Design review of the part built by this model. Coordinates are the model's own, in mm. A direction names the side the tool comes from. Round coordinates to 2 decimals unless told otherwise and drop trailing zeros. Write each loop counter-clockwise with the first axis right and the second up, starting at its lowest first coordinate (ties: lowest second). Pieces come first, ordered by that corner, then holes. Notation, with made-up numbers: (88.25, 48) -> (121.25, 48) arc R19 ccw to (121.25, 57) -> close; hole circle Ø1 at (68, -25). An arc over 180 degrees is marked (long way). One line per question, with ' | ' between items. Start each with the question number.
1) For faces 1 (the flat face through (3.549, 6.034, 2.875)), 2 (the flat face through (5, -2, 0)), 3 (the cylindrical face through (1.322, 4.197, 17.245)), 4 (the cylindrical face through (6.84, -0.9, 18.58)), 5 (the conical face through (-0.158, -7.184, 0.322)), list the 3-axis set-ups (+Z, -Z, +X, -X, +Y, -Y) from which the entire face can be reached by the end or side of a thin tool; tool diameter is ignored.
2) For probe 1 along X at (y, z) = (0, 6.5); probe 2 along X at (y, z) = (-1.25, 7); probe 3 along Y at (x, z) = (-0.75, -2), list the stretches that pass through material, from the lowest coordinate up.
3) Consider section A-A (z = 0.75). Give the boundary of the cut face in (x, y), then the cut area to 3 significant figures.
4) Mouldability with a two-part tool opening along X and no side actions: class faces 6 (the conical face through (0.158, 7.184, 0.322)), 7 (the flat face through (3.45, -6.09, 2.88)), 8 (the flat face through (-2, 3, -8)), 9 (the cylindrical face through (0, -3, -1)) as +X half, -X half, draft (parallel to the pull), parting line (faces both ways), or undercut.
5) Insertion check: pin 1 Ø3 at (x, z) = (-1.5, 16) entering from -Y; pin 2 Ø3.5 at (x, y) = (1, -1.5) entering from +Z; pin 3 Ø4 at (x, z) = (-4.5, 3.5) entering from +Y. Each pin has a flat end and moves straight along its axis. Give the tip position at first contact, or say it passes through.
Autodesk Inventor part; units mm, degrees
ref_plane "ANBAU_XY" through (0, 0, -4) normal (0, 0, 1) x (1, 0, 0)
ref_plane "ANBAU_YZ" through (0, 0, -4) normal (1, 0, 0) x (0, 1, 0)
ref_plane "ANBAU_ZX" through (0, 0, -4) normal (0, 1, 0) x (0, 0, 1)
sketch "Sketch_2" plane through (0, 0, 0) normal (1, 0, 0) x (0, 1, 0)
  line L0 (0, 0) -> (0, 19.9)
  line L1 (0, 19.9) -> (4.3, 19.9)
  line L2 (4.3, 19.9) -> (6.7347, 19.4707)
  arc A0 (6.9, 19.2737) -> (6.7347, 19.4707) centre (6.7, 19.2737) ccw
  line L3 (6.9, 19.2737) -> (6.9, 17.9)
  line L4 (6.9, 17.9) -> (4.7, 17.9)
  arc A1 (4.7, 17.9) -> (4.4, 17.6) centre (4.7, 17.6) ccw
  line L5 (4.4, 17.6) -> (4.4, 16.9)
  line L6 (4.4, 16.9) -> (5.7, 16.9)
  line L7 (5.7, 16.9) -> (5.9, 16.7)
  line L8 (5.9, 16.7) -> (5.9, 16)
  line L9 (5.9, 16) -> (5.8, 15.9)
  line L10 (5.8, 15.9) -> (5.9, 15.8)
  line L11 (5.9, 15.8) -> (5.9, 13.1)
  line L12 (5.9, 13.1) -> (8.4, 13.1)
  line L13 (8.4, 13.1) -> (8.4, 2.4249)
  line L14 (8.4, 2.4249) -> (7, 0)
  line L15 (7, 0) -> (0, 0)
  line L16 (0, 0) -> (0, 19.9)
revolve "Revolution1" add sketch "Sketch_2" angle 360 about axis through (0, 0, 0) along (0, 0, -1)
sketch "Sketch_3" plane through (0, 0, 0) normal (0, 0, 1) x (1, 0, 0)
  line L0 (-14, -14) -> (14, -14)
  line L1 (14, -14) -> (14, 14)
  line L2 (14, 14) -> (-14, 14)
  line L3 (-14, 14) -> (-14, -14)
  line L4 (-7, -4.0415) -> (0, -8.0829)
  line L5 (0, -8.0829) -> (7, -4.0415)
  line L6 (7, -4.0415) -> (7, 4.0415)
  line L7 (7, 4.0415) -> (0, 8.0829)
  line L8 (0, 8.0829) -> (-7, 4.0415)
  line L9 (-7, 4.0415) -> (-7, -4.0415)
extrude "Extrusion1" cut sketch "Sketch_3" along normal blind 13.2
sketch "Sketch_4" plane through (0, 0, 0) normal (1, 0, 0) x (0, 1, 0)
  line L0 (0, -50) -> (0, 50)
  line L1 (6.35, 13.1) -> (6.6964, 12.5)
  line L2 (6.6964, 12.5) -> (6.85, 12.5)
  line L3 (6.85, 12.5) -> (6.85, 4.8)
  line L4 (6.85, 4.8) -> (16.85, 2.1205)
  line L5 (16.85, 2.1205) -> (16.85, 13.1)
  line L6 (16.85, 13.1) -> (6.35, 13.1)
revolve "Revolution2" cut sketch "Sketch_4" angle 360 about axis through (0, 0, -50) along (0, 0, -1)
sketch "Sketch_6" plane through (0, 0, 0) normal (1, 0, 0) x (0, 1, 0)
  line L0 (0, -8) -> (0, 0)
  line L1 (0, 0) -> (4.9889, 0)
  line L2 (4.9889, 0) -> (4.7578, -7.4003)
  line L3 (4.7578, -7.4003) -> (4.1581, -8)
  line L4 (4.1581, -8) -> (0, -8)
  line L5 (0, -8) -> (0, 0)
revolve "Revolution3" add sketch "Sketch_6" angle 360 about axis through (0, 0, -8) along (0, 0, -1)
thread "Thread1"
sketch "Sketch_5" plane through (0, 0, 0) normal (1, 0, 0) x (0, 1, 0)
  line L0 (0, -8) -> (0, 19.9)
  line L1 (0, 19.9) -> (4.3, 19.9)
  arc A0 (4.3, 19.9) -> (4, 19.6) centre (4.3, 19.6) ccw
  line L2 (4, 19.6) -> (4, 1.7)
  line L3 (4, 1.7) -> (3, 1.7)
  line L4 (3, 1.7) -> (3, -4.0389)
  line L5 (3, -4.0389) -> (2.7794, -4)
  line L6 (2.7794, -4) -> (2.7794, -7.5)
  line L7 (2.7794, -7.5) -> (3.2794, -8)
  line L8 (3.2794, -8) -> (0, -8)
  line L9 (0, -8) -> (0, 19.9)
revolve "Revolution4" cut sketch "Sketch_5" angle 360 about axis through (0, 0, -8) along (0, 0, -1)
ref_plane "ANBAU_XY" through (0, 0, -4) normal (0, 0, 1) x (1, 0, 0)
ref_plane "ANBAU_YZ" through (0, 0, -4) normal (1, 0, 0) x (0, 1, 0)
ref_plane "ANBAU_ZX" through (0, 0, -4) normal (0, 1, 0) x (0, 0, 1)
ref_plane "ANBAU_FDT3D_XY" through (0, 0, -4) normal (0, 0, -1) x (1, 0, 0)
ref_plane "ANBAU_FDT3D_YZ" through (0, 0, -4) normal (1, 0, 0) x (0, -1, 0)
ref_plane "ANBAU_FDT3D_ZX" through (0, 0, -4) normal (0, -1, 0) x (0, 0, -1)
ref_plane "ANBAU_STD_XY" through (0, 0, -4) normal (0, 0, 1) x (1, 0, 0)
ref_plane "ANBAU_STD_YZ" through (0, 0, -4) normal (1, 0, 0) x (0, 1, 0)
ref_plane "ANBAU_STD_ZX" through (0, 0, -4) normal (0, 1, 0) x (0, 0, 1)
ref_plane "DROSSEL_XY" through (0, 0, -4) normal (0, 0, -1) x (1, 0, 0)
ref_plane "DROSSEL_YZ" through (0, 0, -4) normal (1, 0, 0) x (0, -1, 0)
ref_plane "DROSSEL_ZX" through (0, 0, -4) normal (0, -1, 0) x (0, 0, -1)
ref_plane "FDT_SCHLAUCH_XY" through (0, 0, 1.7) normal (0, 0, 1) x (1, 0, 0)
ref_plane "FDT_SCHLAUCH_YZ" through (0, 0, 1.7) normal (1, 0, 0) x (0, 1, 0)
ref_plane "FDT_SCHLAUCH_ZX" through (0, 0, 1.7) normal (0, 1, 0) x (0, 0, 1)
ref_plane "TO_CAP_XY" through (0, 0, 19.9) normal (0, 0, 1) x (1, 0, 0)
ref_plane "TO_CAP_YZ" through (0, 0, 19.9) normal (1, 0, 0) x (0, 1, 0)
ref_plane "TO_CAP_ZX" through (0, 0, 19.9) normal (0, 1, 0) x (0, 0, 1)
properties part number "153004 QS-1/8-8"
From the geometry:
1) face 1: +Z, -Z, +X, +Y | face 2: -Z | face 3: none | face 4: +Z | face 5: -Z, -Y
2) probe 1: x = -6.85 to -4, 4 to 6.85 | probe 2: x = -6.73 to -3.8, 3.8 to 6.73 | probe 3: y = -4.87 to -2.9, 2.9 to 4.87
3) outline: (-7, -2.5) arc R7.43 ccw to (-5.66, -4.81) -> (-1.34, -7.31) arc R7.43 ccw to (1.34, -7.31) -> (5.66, -4.81) arc R7.43 ccw to (7, -2.5) -> (7, 2.5) arc R7.43 ccw to (5.66, 4.81) -> (1.34, 7.31) arc R7.43 ccw to (-1.34, 7.31) -> (-5.66, 4.81) arc R7.43 ccw to (-7, 2.5) -> close; hole circle Ø6 at (0, 0) | area: 137 mm2
4) face 6: parting line | face 7: +X half | face 8: draft | face 9: undercut
5) pin 1: stops at y = -5.9 | pin 2: stops at z = 1.7 | pin 3: stops at y = 6.64
